Here's how the part is built. I have some questions about the finished solid (model axes, mm). Round coordinates to 2 decimals unless told otherwise and drop trailing zeros. Loops run counter-clockwise (first coordinate to the right, second up) from the corner with the lowest first, then second, coordinate; pieces in that order, holes last. Notation, with made-up numbers: (45.25, 39) -> (66.25, 39) arc R9 ccw to (66.25, 50) -> close; hole circle Ø2 at (79.25, 26). An arc over 180 degrees is marked (long way). Use CSV: the item, a comma, the result in double quotes. Start each with the question number.
from build123d import *

# Parameters (mm, degrees)
F0_R     = 128.27
F1_DEPTH = 274.32
F6_SIZE  = 5.08


with BuildPart() as f1:
    # F0 (on Front) → F1 (new body)
    with BuildSketch(Plane.XZ):
        Polygon((228.6, -131.982272), (228.6, 131.982272), (0, 263.964543), (-228.6, 131.982272), (-228.6, -131.982272), (0, -263.964543), align=None)
        Circle(F0_R, mode=Mode.SUBTRACT)
    extrude(amount=F1_DEPTH)


with BuildPart() as f2_1:
    # F2: copy of F1
    add(f1.part)

    # F4 (on Top) → F5 (revolve, cut)
    with BuildSketch(Plane.XY):
        Polygon((435.953124, -154.604618), (228.6, -274.32), (435.953124, -274.32), align=None)
        Polygon((228.6, 0), (435.953124, -119.715382), (435.953124, 0), align=None)
    revolve(axis=Axis((0, -137.16, 0), (0, 1, 0)), mode=Mode.SUBTRACT)

    # F6
    f6_edges = [f2_1.edges().sort_by_distance(p)[0] for p in [
        (-128.27, 0, 0),
    ]]
    chamfer(f6_edges, length=F6_SIZE)


solid = f2_1.part
Q1. Will these pins go through, and if not, where does the flat tip stop? pin 1 Ø1.5 at (y, z) = (-123, 199.5) entering from +X; pin 2 Ø1.5 at (x, y) = (-11.5, -63) entering from -Z; pin 3 Ø5 at (x, y) = (18.5, -207.5) entering from -Z.
Q2. If we mould it in two halves opening along X, with no side actions, what happens to faces 1 (the flat face through (98, 0, -98)), 2 (the conical face through (205.707, -4.963, -118.096)), 3 (the cylindrical face through (122.347, -137.815, 38.529))? For each: pulls with the +X half, pulls with the -X half, needs draft (parallel to the pull), parting line crosses it, or undercut.
Q3. I want a section at A-A, the plane y = -75.5. List the corners of the cut face in (x, z) for me, then the cut area to 3 significant figures.
Q4. I need wall thicknesses on line 1 along Z through (x, y) = (0, -122.5); line 2 along Z through (x, y) = (-42, -124); line 3 along X through (y, z) = (-140, 44.5). Which ranges of each line are inside material? Lowest first, please.
Values found:
1,pin 1,"x = 112.95"
1,pin 2,"z = -257.76"
1,pin 3,"z = -254.73"
2,face 1,"needs draft"
2,face 2,"pulls with the +X half"
2,face 3,"undercut"
3,outline,"(-228.6, -131.98) -> (0, -263.96) -> (228.6, -131.98) -> (228.6, 131.98) -> (0, 263.96) -> (-228.6, 131.98) -> close; hole circle Ø256.54 at (0, 0)"
3,area,"129,000 mm2"
4,line 1,"-263.96 to -128.27, 128.27 to 263.96"
4,line 2,"-239.72 to -121.2, 121.2 to 239.72"
4,line 3,"-228.6 to -120.3, 120.3 to 228.6"
